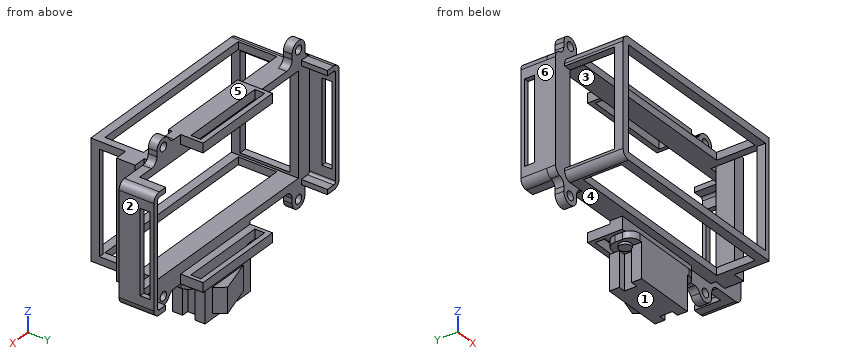
from build123d import *

# Parameters (mm, degrees)
SKETCH_1_W          = 80
SKETCH_1_H          = 47
EXTRUDE_1_DEPTH     = 23.5
EXTRUDE_2_DEPTH     = 3.5
SKETCH_19_R         = 1.75
CUT_EXTRUDE_7_DEPTH = 71.322471515
FILLET_2_R          = 3
SKETCH_3_W          = 85
SKETCH_3_H          = 41
CUT_EXTRUDE_1_DEPTH = 23.5
SKETCH_4_W          = 75
SKETCH_4_H          = 41
CUT_EXTRUDE_2_DEPTH = 4
SKETCH_5_W          = 73
SKETCH_5_H          = 15.5
CUT_EXTRUDE_3_DEPTH = 84.674966388
SKETCH_6_W          = 39
SKETCH_6_H          = 20
CUT_EXTRUDE_4_DEPTH = 4
EXTRUDE_3_REACH     = 89.072
SKETCH_9_W          = 38
SKETCH_9_H          = 5
SKETCH_10_W         = 38
SKETCH_10_H         = 9
EXTRUDE_4_DEPTH     = 3.75
SKETCH_11_W         = 35
SKETCH_11_H         = 4
CUT_EXTRUDE_5_DEPTH = 3.75
FILLET_3_R          = 3
FILLET_4_R          = 3
EXTRUDE_START       = 10.5
EXTRUDE_5_DEPTH     = 10.5
SKETCH_13_W         = 33.381049962
SKETCH_13_H         = 4
CUT_EXTRUDE_6_DEPTH = 113.838380057
SKETCH_14_W         = 47
SKETCH_14_H         = 7.5
EXTRUDE_6_DEPTH     = 5
SKETCH_15_W         = 35
SKETCH_15_H         = 11
EXTRUDE_7_DEPTH     = 2.75
SKETCH_16_W         = 25
SKETCH_16_H         = 13
EXTRUDE_8_DEPTH     = 14
SKETCH_21_W         = 2.8
SKETCH_21_H         = 5
CUT_EXTRUDE_8_DEPTH = 14
SKETCH_20_R         = 2.35
EXTRUDE_10_DEPTH    = 1
FILLET_5_R          = 4
EXTRUDE_START_2     = -2
EXTRUDE_9_DEPTH     = 10


with BuildPart() as part:
    # 草图1 → 凸台-拉伸1 (new body)
    with BuildSketch(Plane(origin=(0, 0, 0), x_dir=(1, 0, 0), z_dir=(0, 1, 0))):
        Rectangle(SKETCH_1_W, SKETCH_1_H)
    extrude(amount=EXTRUDE_1_DEPTH)

    # 草图2 → 凸台-拉伸2 (add)
    with BuildSketch(Plane(origin=(0, 23.5, 0), x_dir=(1, 0, 0), z_dir=(0, 1, 0))):
        with BuildLine():
            Line((-10.5, -28.5), (33.5, -28.5))
            ThreePointArc((33.5, -28.5), (37, -32), (40.5, -28.5))
            Line((40.5, -28.5), (40.5, -23.5))
            Line((40.5, -23.5), (56.5, -23.5))
            Line((56.5, -23.5), (56.5, 23.5))
            Line((56.5, 23.5), (40.5, 23.5))
            Line((40.5, 23.5), (40.5, 28.5))
            ThreePointArc((40.5, 28.5), (37, 32), (33.5, 28.5))
            Line((33.5, 28.5), (-10.5, 28.5))
            Line((-10.5, 28.5), (-10.5, 23.5))
            Line((-10.5, 23.5), (-33.5, 23.5))
            Line((-33.5, 23.5), (-33.5, 28.5))
            ThreePointArc((-33.5, 28.5), (-37, 32), (-40.5, 28.5))
            Line((-40.5, 28.5), (-40.5, 23.5))
            Line((-40.5, 23.5), (-45, 23.5))
            Line((-45, 23.5), (-45, -23.5))
            Line((-45, -23.5), (-40.5, -23.5))
            Line((-40.5, -23.5), (-40.5, -28.5))
            ThreePointArc((-40.5, -28.5), (-37, -32), (-33.5, -28.5))
            Line((-33.5, -28.5), (-33.5, -23.5))
            Line((-33.5, -23.5), (-10.5, -23.5))
            Line((-10.5, -23.5), (-10.5, -28.5))
        make_face()
    extrude(amount=EXTRUDE_2_DEPTH)

    # 草图19 → 切除-拉伸7 (cut, through all)
    with BuildSketch(Plane(origin=(0, 27, 0), x_dir=(1, 0, 0), z_dir=(0, 1, 0))):
        with Locations(Location((-37, 28.5, 0), (0, 0, 270))):
            Circle(SKETCH_19_R)
        with Locations(Location((37, 28.5, 0), (0, 0, 270))):
            Circle(SKETCH_19_R)
        with Locations(Location((37, -28.5, 0), (0, 0, 270))):
            Circle(SKETCH_19_R)
        with Locations(Location((-37, -28.5, 0), (0, 0, 270))):
            Circle(SKETCH_19_R)
    extrude(amount=-CUT_EXTRUDE_7_DEPTH, mode=Mode.SUBTRACT)

    # 圆角2
    fillet_2_edges = [part.edges().sort_by_distance(p)[0] for p in [
        (-40, 11.75, -23.5),
        (-40, 11.75, 23.5),
    ]]
    fillet(fillet_2_edges, radius=FILLET_2_R)

    # 草图3 → 切除-拉伸1 (cut)
    with BuildSketch(Plane(origin=(0, 27, 0), x_dir=(1, 0, 0), z_dir=(0, 1, 0))):
        with Locations((5.5, 0)):
            Rectangle(SKETCH_3_W, SKETCH_3_H)
    extrude(amount=-CUT_EXTRUDE_1_DEPTH, mode=Mode.SUBTRACT)

    # 草图4 → 切除-拉伸2 (cut)
    with BuildSketch(Plane.XZ):
        with Locations((0.5, 0)):
            Rectangle(SKETCH_4_W, SKETCH_4_H)
    extrude(amount=-CUT_EXTRUDE_2_DEPTH, mode=Mode.SUBTRACT)

    # 草图5 → 切除-拉伸3 (cut, through all)
    with BuildSketch(Plane.XY.offset(23.5)):
        with Locations((0.5, 11.25)):
            Rectangle(SKETCH_5_W, SKETCH_5_H)
    extrude(amount=-CUT_EXTRUDE_3_DEPTH, mode=Mode.SUBTRACT)

    # 草图6 → 切除-拉伸4 (cut)
    with BuildSketch(Plane.ZY.offset(40)):
        with Locations((0, 13.5)):
            Rectangle(SKETCH_6_W, SKETCH_6_H)
    extrude(amount=-CUT_EXTRUDE_4_DEPTH, mode=Mode.SUBTRACT)

    # 草图9 → 凸台-拉伸3 (add, up to next)
    with BuildSketch(Plane.XY.offset(28.5), mode=Mode.PRIVATE) as extrude_3_sk1:
        with Locations((8.5, 24.5)):
            Rectangle(SKETCH_9_W, SKETCH_9_H)
    extrude_3_tool1 = extrude(extrude_3_sk1.sketch, amount=-EXTRUDE_3_REACH, mode=Mode.PRIVATE) - part.part
    extrude_3 = extrude_3_tool1.solids().sort_by_distance((8.5, 24.5, 28.5))[0]
    add(extrude_3)

    # 草图10 → 凸台-拉伸4 (add)
    with BuildSketch(Plane.XY.offset(28.5)):
        with Locations((8.5, 31.5)):
            Rectangle(SKETCH_10_W, SKETCH_10_H)
    extrude_4 = extrude(amount=-EXTRUDE_4_DEPTH)

    # 草图11 → 切除-拉伸5 (cut)
    with BuildSketch(Plane.XY.offset(28.5)):
        with Locations((8.5, 32)):
            Rectangle(SKETCH_11_W, SKETCH_11_H)
    cut_extrude_5 = extrude(amount=-CUT_EXTRUDE_5_DEPTH, mode=Mode.SUBTRACT)

    # 镜向1: 凸台-拉伸3, 凸台-拉伸4, 切除-拉伸5 across plane
    add(extrude_3.mirror(Plane.XY))
    add(extrude_4.mirror(Plane.XY))
    add(cut_extrude_5.mirror(Plane.XY), mode=Mode.SUBTRACT)

    # 圆角3
    fillet_3_edges = [part.edges().sort_by_distance(p)[0] for p in [
        (33.5, 25.25, 28.5),
        (-40.5, 25.25, 23.5),
        (40.5, 25.25, -23.5),
        (33.5, 25.25, -28.5),
        (-33.5, 25.25, -23.5),
        (-33.5, 25.25, 23.5),
        (40.5, 25.25, 23.5),
        (-40.5, 25.25, -23.5),
    ]]
    fillet(fillet_3_edges, radius=FILLET_3_R)

    # 圆角4
    fillet_4_edges = [part.edges().sort_by_distance(p)[0] for p in [
        (56.5, 25.25, 23.5),
        (56.5, 25.25, -23.5),
        (-45, 25.25, -23.5),
        (-45, 25.25, 23.5),
    ]]
    fillet(fillet_4_edges, radius=FILLET_4_R)

    # 草图12 → 凸台-拉伸5 (add)
    with BuildSketch(Plane(origin=(0, 27, 0), x_dir=(1, 0, 0), z_dir=(0, 1, 0)).offset(EXTRUDE_START)):
        with BuildLine():
            Line((-45, 20.690524981), (-45, -20.690524981))
            ThreePointArc((-45, -20.690524981), (-44.121320344, -22.811845324), (-42, -23.690524981))
            Line((-42, -23.690524981), (-38.5, -23.690524981))
            Line((-38.5, -23.690524981), (-38.5, -21.690524981))
            Line((-38.5, -21.690524981), (-42, -21.690524981))
            ThreePointArc((-42, -21.690524981), (-42.707106781, -21.397631762), (-43, -20.690524981))
            Line((-43, -20.690524981), (-43, 20.690524981))
            ThreePointArc((-43, 20.690524981), (-42.707106781, 21.397631762), (-42, 21.690524981))
            Line((-42, 21.690524981), (-38.5, 21.690524981))
            Line((-38.5, 21.690524981), (-38.5, 23.690524981))
            Line((-38.5, 23.690524981), (-42, 23.690524981))
            ThreePointArc((-42, 23.690524981), (-44.121320344, 22.811845324), (-45, 20.690524981))
        make_face()
        with BuildLine():
            Line((53.5, 23.5), (50, 23.5))
            Line((50, 23.5), (50, 21.5))
            Line((50, 21.5), (53.5, 21.5))
            ThreePointArc((53.5, 21.5), (54.207106781, 21.207106781), (54.5, 20.5))
            Line((54.5, 20.5), (54.5, -20.5))
            ThreePointArc((54.5, -20.5), (54.207106781, -21.207106781), (53.5, -21.5))
            Line((53.5, -21.5), (50, -21.5))
            Line((50, -21.5), (50, -23.5))
            Line((50, -23.5), (53.5, -23.5))
            ThreePointArc((53.5, -23.5), (55.621320344, -22.621320344), (56.5, -20.5))
            Line((56.5, -20.5), (56.5, 20.5))
            ThreePointArc((56.5, 20.5), (55.621320344, 22.621320344), (53.5, 23.5))
        make_face()
    extrude(amount=-EXTRUDE_5_DEPTH)

    # 草图13 → 切除-拉伸6 (cut, through all)
    with BuildSketch(Plane.ZY.offset(45)):
        with Locations((0, 34)):
            Rectangle(SKETCH_13_W, SKETCH_13_H)
    extrude(amount=-CUT_EXTRUDE_6_DEPTH, mode=Mode.SUBTRACT)

    # 草图14 → 凸台-拉伸6 (add)
    with BuildSketch(Plane(origin=(40, 0, 0), x_dir=(0, 0, -1), z_dir=(1, 0, 0))):
        with Locations((0, 17.75)):
            Rectangle(SKETCH_14_W, SKETCH_14_H)
    extrude(amount=EXTRUDE_6_DEPTH)

    # 草图15 → 凸台-拉伸7 (add)
    with BuildSketch(Plane.XY.offset(-28.5)):
        with Locations((8.5, 24.5)):
            Rectangle(SKETCH_15_W, SKETCH_15_H)
    extrude(amount=-EXTRUDE_7_DEPTH)

    # 草图16 → 凸台-拉伸8 (add)
    with BuildSketch(Plane(origin=(0, 0, -31.25), x_dir=(-1, 0, 0), z_dir=(0, 0, -1))):
        with Locations((-8.5, 25.5)):
            Rectangle(SKETCH_16_W, SKETCH_16_H)
    extrude(amount=EXTRUDE_8_DEPTH)

    # 草图21 → 切除-拉伸8 (cut)
    with BuildSketch(Plane(origin=(0, 0, -45.25), x_dir=(-1, 0, 0), z_dir=(0, 0, -1))):
        with Locations((-19.6, 25.5)):
            Rectangle(SKETCH_21_W, SKETCH_21_H)
        with Locations((2.6, 25.5)):
            Rectangle(SKETCH_21_W, SKETCH_21_H)
    extrude(amount=-CUT_EXTRUDE_8_DEPTH, mode=Mode.SUBTRACT)

    # 草图20 → 凸台-拉伸10 (add)
    with BuildSketch(Plane(origin=(0, 0, -31.25), x_dir=(-1, 0, 0), z_dir=(0, 0, -1))):
        with Locations((-22.5, 24.5)):
            Circle(SKETCH_20_R)
        with Locations((5.5, 24.5)):
            Circle(SKETCH_20_R)
    extrude(amount=EXTRUDE_10_DEPTH)

    # 圆角5
    # the kernel refuses this fillet: 4 mm, written as the material it takes off along each edge
    with BuildSketch(Plane(origin=(26, 19, -28.5), x_dir=(-1, 0, 0), z_dir=(0, 0, -1)), Plane(origin=(-9, 30, -28.5), x_dir=(1, 0, 0), z_dir=(0, 0, -1))) as fillet_5_piece_1:
        with BuildLine():
            CenterArc((FILLET_5_R, FILLET_5_R), FILLET_5_R, 180, 90)
            Line((0, FILLET_5_R), (0, 0))
            Line((0, 0), (FILLET_5_R, 0))
        make_face()
    extrude(amount=12.75, mode=Mode.SUBTRACT)
    with BuildSketch(Plane(origin=(26, 30, -28.5), x_dir=(-1, 0, 0), z_dir=(0, 0, -1)), Plane(origin=(-9, 19, -28.5), x_dir=(1, 0, 0), z_dir=(0, 0, -1))) as fillet_5_piece_2:
        with BuildLine():
            CenterArc((FILLET_5_R, -FILLET_5_R), FILLET_5_R, 90, 90)
            Line((0, -FILLET_5_R), (0, 0))
            Line((0, 0), (FILLET_5_R, 0))
        make_face()
    extrude(amount=12.75, mode=Mode.SUBTRACT)

    # 草图17 → 凸台-拉伸9 (add)
    with BuildSketch(Plane(origin=(0, 0, -45.25), x_dir=(-1, 0, 0), z_dir=(0, 0, -1)).offset(EXTRUDE_START_2)):
        Polygon((-17, 32), (-14, 36), (0, 32), align=None)
    extrude(amount=-EXTRUDE_9_DEPTH)


solid = part.part
Work out the finished part from the listing and answer in its coordinate system (mm). Face numbers are marked on the shaded views. A direction names the side the tool comes from. Coordinates: 2 decimals unless noted, no trailing zeros. Order: outer loops, then holes, each group sorted by start corner. A loop starts at its lowest first (then second) coordinate and runs counter-clockwise, first axis right, second up. Notation, with made-up numbers: (81.5, 20) - (140.5, 20) arc R27 cw to (140.5, 39) - close; hole circle Ø10 at (-23, -2). An arc over 180 degrees is marked (long way). Put each result on its own line as item: value. Start each with the question number.
1) Find section C-C (x = -15). Give the vertices of the cut face in (y, z).
2) For a pull along Z with two mould halves and no side action, classify the marked faces 1, 2 and 3 as released by +Z, released by -Z, zero draft, split by the parting line, or undercut.
3) Find the intervals of material crossed by line 1 (Y direction, x = 14, z = 22.5); line 2 (Y direction, x = 17.5, z = 26); line 3 (X direction, y = 30, z = 14.5), in increasing order. Write a range as from..to.
4) Find section B-B (y = 11.5). Give the vertices of the cut face in (x, z).
5) Find section A-A (z = 7.5). State how many separate pieces and enclosed holes the cut face has, plus the area to 3 significant figures.
6) Find section D-D (y = 16.5). Give the vertices of the cut face in (x, z), plus the area to 3 significant figures.
7) Flat-ended cylindrical pins translate along their axes: pin 1 (2 mm diameter, centred on y = 24.5, z = -29.5, fed in from +X); pin 2 (3 mm diameter, centred on y = 29.5, z = -41, fed in from +X); pin 3 (1.6 mm diameter, centred on x = 39.5, z = -0.5, fed in from +Y); pin 4 (2 mm diameter, centred on y = 12, z = 16.5, fed in from -X). Find the tip coordinate at first contact, or state that the pin passes through.
8) For the marked faces 4, 5 and 6, determine the directions among +Z, -Z, +X, -X, +Y, -Y from which every point of the face is accessible in a straight line to the end or side of a thin tool.
Results list:
1. outline: (0, -23.5) - (3.5, -23.5) - (3.5, -20.5) - (0, -20.5) - close; (0, 20.5) - (3.5, 20.5) - (3.5, 23.5) - (0, 23.5) - close; (19, -23.5) - (27, -23.5) - (27, -20.5) - (19, -20.5) - close; (19, 20.5) - (27, 20.5) - (27, 23.5) - (19, 23.5) - close
2. face 1: released by -Z
2. face 2: zero draft
2. face 3: undercut
3. line 1: y = 0..3.5, 19..27
3. line 2: y = 22..30, 34..36
3. line 3: x = -45..-43, 54.5..56.5
4. outline: (-40, -20.5) arc R3 ccw to (-37, -23.5) - (-36, -23.5) - (-36, -20.5) - (-37, -20.5) - (-37, -19.5) - (-40, -19.5) - close; (-40, 19.5) - (-37, 19.5) - (-37, 20.5) - (-36, 20.5) - (-36, 23.5) - (-37, 23.5) arc R3 ccw to (-40, 20.5) - close; (37, -23.5) - (40, -23.5) - (40, -20.5) - (37, -20.5) - close; (37, 20.5) - (40, 20.5) - (40, 23.5) - (37, 23.5) - close
5. separate pieces: 7
5. enclosed holes: 0
5. area: 139 mm^2
6. outline: (-40, -20.5) arc R3 ccw to (-37, -23.5) - (-36, -23.5) - (-36, -20.5) - (-37, -20.5) - (-37, -19.5) - (-40, -19.5) - close; (-40, 19.5) - (-37, 19.5) - (-37, 20.5) - (-36, 20.5) - (-36, 23.5) - (-37, 23.5) arc R3 ccw to (-40, 20.5) - close; (37, -23.5) - (45, -23.5) - (45, 23.5) - (37, 23.5) - (37, 20.5) - (40, 20.5) - (40, -20.5) - (37, -20.5) - close
6. area: 279 mm^2
7. pin 1: stops at x = 40.5
7. pin 2: stops at x = 21
7. pin 3: stops at y = 21.5
7. pin 4: passes through
8. face 4: -Y
8. face 5: +Z, +Y, -Y
8. face 6: +Z, -Z, -X, +Y, -Y
